```python
from build123d import *

# Parameters (mm, degrees)
SKETCH1_W           = 16
SKETCH1_H           = 13.83
BOSS_EXTRUDE1_DEPTH = 25
SKETCH2_W           = 1
SKETCH2_H           = 1.15
BOSS_EXTRUDE3_DEPTH = 16.73
SKETCH3_W           = 1.4
SKETCH3_H           = 1.31
SKETCH3_W_2         = 1.3
CUT_EXTRUDE1_DEPTH  = 23.6
SKETCH5_W           = 16
SKETCH5_H           = 13.83
CUT_EXTRUDE2_DEPTH  = 10


with BuildPart() as part:
    # Sketch1 → Boss-Extrude1 (new body)
    with BuildSketch(Plane(origin=(0, 0, 0), x_dir=(1, 0, 0), z_dir=(0, 1, 0))):
        with Locations((6.25, 4.915)):
            Rectangle(SKETCH1_W, SKETCH1_H)
        Polygon((0, 0), (0, 7.25), (2.85, 7.25), (2.85, 8.52), (4.25, 8.52), (4.25, 9.83), (8.25, 9.83), (8.25, 8.52), (9.55, 8.52), (9.55, 7.25), (12.5, 7.25), (12.5, 0), align=None, mode=Mode.SUBTRACT)
    extrude(amount=BOSS_EXTRUDE1_DEPTH)

    # Sketch2 → Boss-Extrude3 (add)
    with BuildSketch(Plane.XZ):
        with Locations((12, -6.675)):
            Rectangle(SKETCH2_W, SKETCH2_H)
        with Locations((0.5, -6.675)):
            Rectangle(SKETCH2_W, SKETCH2_H)
    extrude(amount=-BOSS_EXTRUDE3_DEPTH)

    # Sketch3 → Cut-Extrude1 (cut)
    with BuildSketch(Plane.XZ):
        with Locations((3.55, -9.175)):
            Rectangle(SKETCH3_W, SKETCH3_H)
        with Locations((8.9, -9.175)):
            Rectangle(SKETCH3_W_2, SKETCH3_H)
    extrude(amount=-CUT_EXTRUDE1_DEPTH, mode=Mode.SUBTRACT)

    # Sketch5 → Cut-Extrude2 (cut)
    with BuildSketch(Plane.XZ):
        with Locations((6.25, -4.915)):
            Rectangle(SKETCH5_W, SKETCH5_H)
    extrude(amount=-CUT_EXTRUDE2_DEPTH, mode=Mode.SUBTRACT)


solid = part.part
```
The listing builds one solid part. Answer for the finished solid, in the listing's coordinates (mm). A direction names the side the tool comes from. Coordinates: 2 decimals unless noted, no trailing zeros. Write each loop counter-clockwise with the first axis right and the second up, starting at its lowest first coordinate (ties: lowest second). Pieces come first, ordered by that corner, then holes. Notation, with made-up numbers: (7, 29) - (25, 29) arc R16 cw to (25, 56) - close; hole circle Ø4 at (46, -4). An arc over 180 degrees is marked (long way). Return JSON: item names as keys, results as strings. Group by question number.
Q1. For a pull along X with two mould halves and no side action, classify faces 1 (the flat face through (6, 17, -11.83)), 2 (the flat face through (14.25, 17, -5)), 3 (the flat face through (6, 17, -9.83)), 4 (the flat face through (-1.75, 17, -5)) as +X half, -X half, draft (parallel to the pull), parting line (faces both ways), or undercut.
Q2. The part is cut by section D-D on x = 1.75. Write down the section's boundary in (y, z), and give its area (3 significant figures).
Q3. The part is cut by section B-B on x = 9.25. Write down the section's boundary in (y, z).
Q4. The part is cut by section A-A on z = -6.75. Write down the section's boundary in (x, y).
Q5. The part is cut by section C-C on y = 19. Write down the section's boundary in (x, z).
Q6. Which of the six approach directions +Z, -Z, +X, -X, +Y, -Y give full straight-line access (tool end or side, diameter ignored) to faces 5 (the flat face through (10, 25, -8)), 6 (the flat face through (2, 17, -7.25)), 7 (the flat face through (9.55, 17, -9)), 8 (the flat face through (0.5, 13.3, -6.1))?
Q7. Find the intervals of material crossed by line 1 along X through (y, z) = (18, -1); line 2 along Z through (x, y) = (7, 23.5); line 3 along X through (y, z) = (11, -9.75), in increasing order. Write a range as [from, to].
Evaluation:
{
 "1": {"face 1": "draft", "face 2": "+X half", "face 3": "undercut", "face 4": "-X half"},
 "2": {"outline": "(10, -11.83) - (25, -11.83) - (25, -7.25) - (10, -7.25) - close; (10, 0) - (25, 0) - (25, 2) - (10, 2) - close", "area": "98.7 mm2"},
 "3": {"outline": "(10, -11.83) - (25, -11.83) - (25, -8.52) - (23.6, -8.52) - (23.6, -9.83) - (10, -9.83) - close; (10, 0) - (25, 0) - (25, 2) - (10, 2) - close"},
 "4": {"outline": "(-1.75, 10) - (1, 10) - (1, 16.73) - (0, 16.73) - (0, 25) - (-1.75, 25) - close; (11.5, 10) - (14.25, 10) - (14.25, 25) - (12.5, 25) - (12.5, 16.73) - (11.5, 16.73) - close"},
 "5": {"outline": "(-1.75, -11.83) - (14.25, -11.83) - (14.25, 2) - (-1.75, 2) - close; hole (0, -7.25) - (2.85, -7.25) - (2.85, -9.83) - (9.55, -9.83) - (9.55, -7.25) - (12.5, -7.25) - (12.5, 0) - (0, 0) - close"},
 "6": {"face 5": "+Z, -Z, +X, -X, +Y", "face 6": "+Y", "face 7": "-Y", "face 8": "+Y, -Y"},
 "7": {"line 1": "x = [-1.75, 0], [12.5, 14.25]", "line 2": "z = [-11.83, -9.83], [0, 2]", "line 3": "x = [-1.75, 2.85], [9.55, 14.25]"}
}
